Can you work these out from the model? Positions are in its coordinate system, mm. Give positions to 0.01 mm unless a question says otherwise; leave off trailing zeros. Loops run counter-clockwise (first coordinate to the right, second up) from the corner with the lowest first, then second, coordinate; pieces in that order, holes last. Notation, with made-up numbers: (-22.5, -23) - (-18.5, -23) arc R13 ccw to (-18.5, -16) - close; hole circle Ø2 at (8, -16.5). An arc over 180 degrees is marked (long way). Answer in a Markdown table with one row per item.
from build123d import *

# Parameters (mm, degrees)
EXTRUDE_THIN1_DEPTH = 285.75
FILLET1_R           = 1.016


with BuildPart() as part:
    # Sketch1 → Extrude-Thin1 (new body)
    with BuildSketch(Plane.XY):
        with BuildLine():
            Line((0, 3.175), (0, 0))
            Line((0, 0), (-7.9375, 0))
            Line((-7.9375, 0), (-7.9375, 2.38125))
            ThreePointArc((-7.9375, 2.38125), (-19.045912437, 5.99541523), (-27.361917214, 14.199260776))
            ThreePointArc((-27.361917214, 14.199260776), (-27.934001551, 21.541515485), (-22.225, 26.19375))
            Line((-22.225, 26.19375), (-22.225, 28.575))
            Line((-22.225, 28.575), (0, 26.9875))
            Line((0, 26.9875), (-0.226785714, 23.8125))
            Line((-0.226785714, 23.8125), (-1.240203753, 23.884887003))
            Line((-1.240203753, 23.884887003), (-1.085805042, 26.046468964))
            Line((-1.085805042, 26.046468964), (-21.209, 27.483840032))
            Line((-21.209, 27.483840032), (-21.209, 25.314485679))
            ThreePointArc((-21.209, 25.314485679), (-26.827226174, 21.514111333), (-26.50119181, 14.739082765))
            ThreePointArc((-26.50119181, 14.739082765), (-18.11648679, 6.624447995), (-6.9215, 3.334638499))
            Line((-6.9215, 3.334638499), (-6.9215, 1.016))
            Line((-6.9215, 1.016), (-1.016, 1.016))
            Line((-1.016, 1.016), (-1.016, 3.175))
            Line((-1.016, 3.175), (0, 3.175))
        make_face()
    extrude(amount=-EXTRUDE_THIN1_DEPTH)

    # Fillet1
    fillet1_edges = [part.edges().sort_by_distance(p)[0] for p in [
        (-21.209, 25.314485679, -142.875),
        (-6.9215, 3.334638499, -142.875),
        (0, 0, -142.875),
        (-7.9375, 0, -142.875),
        (-22.225, 28.575, -142.875),
        (0, 26.9875, -142.875),
    ]]
    fillet(fillet1_edges, radius=FILLET1_R)


solid = part.part
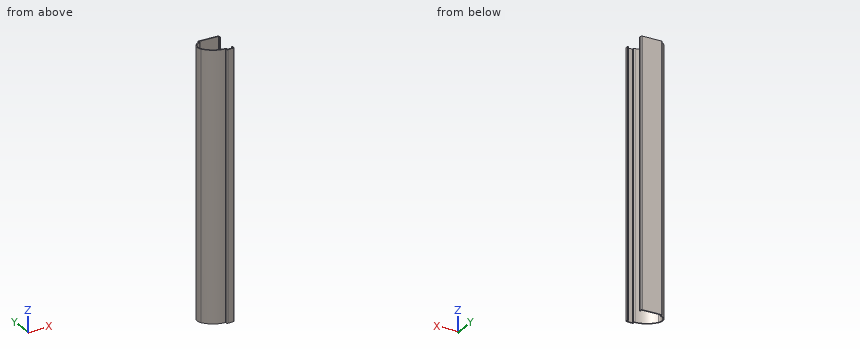
Q1. Imagine slicing it at B-B, the plane z = -208. Write out the boundary of the cut face in (x, y) (1 decimal), and give its area (3 significant figures).
Checked values:
| item | result |
|---|---|
| outline | (-27.4, 14.2) arc R25.4 ccw to (-7.9, 2.4) - (-7.9, 1) arc R1 ccw to (-6.9, 0) - (-1, 0) arc R1 ccw to (0, 1) - (0, 3.2) - (-1, 3.2) - (-1, 1) - (-6.9, 1) - (-6.9, 2.4) arc R1 ccw to (-7.9, 3.4) arc R24.4 cw to (-26.5, 14.7) arc R6.9 cw to (-22, 25.2) arc R1 ccw to (-21.2, 26.2) - (-21.2, 27.5) - (-1.1, 26) - (-1.2, 23.9) - (-0.2, 23.8) - (-0.1, 26) arc R1 ccw to (-1, 27.1) - (-21.1, 28.5) arc R1 ccw to (-22.2, 27.5) - (-22.2, 26.2) arc R7.9 ccw to start |
| area | 76.4 mm² |
Q2. For pin 1 (1.4 mm diameter, centred on y = 27, z = -112, fed in from +X); pin 2 (6 mm diameter, centred on x = -11.5, z = -81, fed in from -Y); pin 3 (6 mm diameter, centred on y = 8, z = -31.5, fed in from -X); pin 4 (1.5 mm diameter, centred on y = 2, z = -80, fed in from +X), each with a flat end and sliding along its axis, tell me the tip position at first contact or that it passes through.
Checked values:
| item | result |
|---|---|
| pin 1 | stops at x = -0.1 |
| pin 2 | stops at y = 2.43 |
| pin 3 | stops at x = -24.99 |
| pin 4 | stops at x = 0 |
Q3. If I drill on line 1 (X direction, y = 1.5, z = -180); line 2 (Y direction, x = -12.5, z = -189); line 3 (Y direction, x = -20.25, z = -249.5), over which ranges is the centre line in solid material (lowest first)? Write a range as [from, to].
Checked values:
| item | result |
|---|---|
| line 1 | x = [-7.94, -6.92], [-1.02, 0] |
| line 2 | y = [3.18, 4.24], [26.86, 27.88] |
| line 3 | y = [6.78, 8.02], [27.42, 28.43] |
Q4. Imagine slicing it at C-C, the plane y = 17.25. Write out the boundary of the cut face in (x, z), and give its area (3 significant figures).
Checked values:
| item | result |
|---|---|
| outline | (-28.49, -285.75) - (-27.46, -285.75) - (-27.46, 0) - (-28.49, 0) - close |
| area | 294 mm² |
Q5. Imagine slicing it at A-A, the plane x = -17. Write out the boundary of the cut face in (y, z), and give its area (3 significant figures).
Checked values:
| item | result |
|---|---|
| outline | (4.88, -285.75) - (6.01, -285.75) - (6.01, 0) - (4.88, 0) - close; (27.18, -285.75) - (28.2, -285.75) - (28.2, 0) - (27.18, 0) - close |
| area | 616 mm² |
